The drawing under review shows one solid part. Ordinate dimensions are in mm from its lowest x, y, z. A direction names the side the tool comes from. Coordinates: 2 decimals unless noted, no trailing zeros. Write each loop counter-clockwise with the first axis right and the second up, starting at its lowest first coordinate (ties: lowest second). Pieces come first, ordered by that corner, then holes.
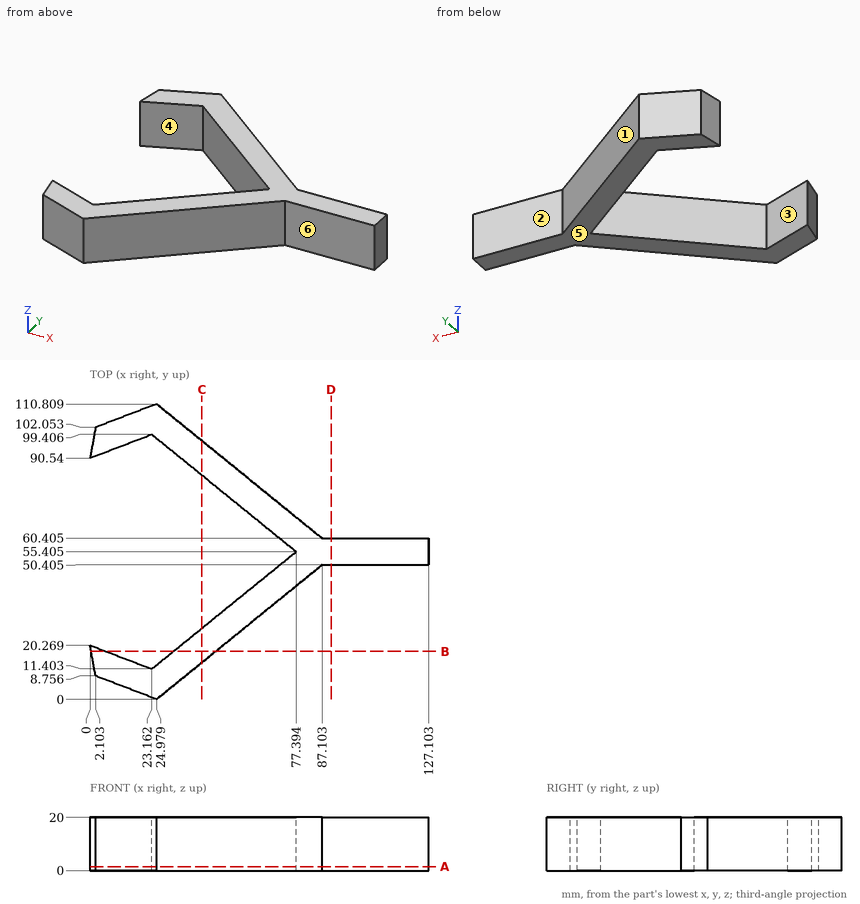
Q1. Clearance check with flat-ended pins moving along their axes: pin 1 Ø2 at (x, z) = (45, 6) entering from +Y; pin 2 Ø4 at (x, z) = (67.5, 15.5) entering from -Y; pin 3 Ø4 at (y, z) = (68, 13) entering from +X (1 decimal). State where each tip first meets the part, or that it passes through.
Ans:
pin 1: stops at y = 95.38
pin 2: stops at y = 32.88
pin 3: stops at x = 80.2
Q2. Add section D-D (x = 90.5). State the section outline as (y, z) points (1 decimal), then the cut area to 3 significant figures.
Ans:
outline: (50.4, 0) - (60.4, 0) - (60.4, 20) - (50.4, 20) - close
area: 200 mm2
Q3. Draft analysis for pull direction X (two halves, no side actions). For the marked faces 1, 2 and 3, state which applies: +X half, -X half, draft (parallel to the pull), parting line (faces both ways), or undercut.
Ans:
face 1: +X half
face 2: draft
face 3: undercut
Q4. Add section B-B (y = 18). State the section outline as (x, z) points (1 decimal).
Ans:
outline: (0.4, 0) - (5.9, 0) - (5.9, 20) - (0.4, 20) - close; (31.3, 0) - (47.2, 0) - (47.2, 20) - (31.3, 20) - close
Q5. Add section C-C (x = 42). State the section outline as (y, z) points, then the cut area to 3 significant figures.
Ans:
outline: (13.81, 0) - (26.69, 0) - (26.69, 20) - (13.81, 20) - close; (84.12, 0) - (97, 0) - (97, 20) - (84.12, 20) - close
area: 515 mm2
Q6. For probe 1 along Y at (x, z) = (98, 6.75) (1 decimal); probe 2 along Y at (x, z) = (69, 5.75) (1 decimal); probe 3 along Y at (x, z) = (8, 13.75), list the stretches that pass through material, from the lowest coordinate up.
Ans:
probe 1: y = 50.4 to 60.4
probe 2: y = 35.7 to 48.6, 62.2 to 75.1
probe 3: y = 6.5 to 17.21, 93.6 to 104.31
Q7. Tool access review of the marked faces 4, 5 and 6: name each direction out of +Z, -Z, +X, -X, +Y, -Y from which nothing blocks a thin tool from reaching the whole face with its end or side.
Ans:
face 4: +Z, -Z
face 5: -Z, +X, -X, +Y, -Y
face 6: +Z, -Z, +X, -Y
Q8. Add section A-A (z = 1.5). State the section outline as (x, y) points (1 decimal), then the cut area to 3 significant figures.
Ans:
outline: (0, 20.3) - (2.1, 8.8) - (25, 0) - (87.1, 50.4) - (127.1, 50.4) - (127.1, 60.4) - (87.1, 60.4) - (25, 110.8) - (2.1, 102.1) - (0, 90.5) - (23.2, 99.4) - (77.4, 55.4) - (23.2, 11.4) - close
area: 2,440 mm2
